```python
from build123d import *

# Parameters (mm, degrees)
F0_R     = 3
F0_W     = 10
F0_H     = 12
F1_DEPTH = 17
F2_R     = 3
F3_DEPTH = 12.5
F4_R     = 4


with BuildPart() as f1:
    # F0 (on Top) → F1 (new body)
    with BuildSketch(Plane.XY):
        with BuildLine():
            ThreePointArc((-12, -4), (-18, 2.0000000001), (-11.9999999997, 8))
            Line((-11.9999999997, 8), (-37.5, 8))
            Line((-37.5, 8), (-37.5, -4))
            Line((-37.5, -4), (-12, -4))
        make_face()
        with BuildLine():
            ThreePointArc((-6, 2), (-7.7573593128, 6.242640687), (-11.9999999997, 8))
            ThreePointArc((-11.9999999997, 8), (-18, 2.0000000001), (-12, -4))
            ThreePointArc((-12, -4), (-7.7573593129, -2.2426406871), (-6, 2))
        make_face()
        with Locations((-12, 2)):
            Circle(F0_R, mode=Mode.SUBTRACT)
        with Locations((-12, 2)):
            Circle(F0_R)
        with BuildLine():
            ThreePointArc((12, -4), (6, 2), (12, 8))
            Line((12, 8), (-11.9999999997, 8))
            ThreePointArc((-11.9999999997, 8), (-7.7573593128, 6.242640687), (-6, 2))
            ThreePointArc((-6, 2), (-7.7573593129, -2.2426406871), (-12, -4))
            Line((-12, -4), (12, -4))
        make_face()
        with BuildLine():
            ThreePointArc((12, -4), (16.2426406871, -2.2426406871), (18, 2))
            ThreePointArc((18, 2), (16.2426406871, 6.2426406871), (12, 8))
            ThreePointArc((12, 8), (6, 2), (12, -4))
        make_face()
        with Locations((12, 2)):
            Circle(F0_R, mode=Mode.SUBTRACT)
        with Locations((12, 2)):
            Circle(F0_R)
        with BuildLine():
            ThreePointArc((12, 8), (16.2426406871, 6.2426406871), (18, 2))
            ThreePointArc((18, 2), (16.2426406871, -2.2426406871), (12, -4))
            Line((12, -4), (37.5, -4))
            Line((37.5, -4), (37.5, 8))
            Line((37.5, 8), (12, 8))
        make_face()
        with Locations((-42.5, 2)):
            Rectangle(F0_W, F0_H)
        with Locations((42.5, 2)):
            Rectangle(F0_W, F0_H)
    extrude(amount=F1_DEPTH)

    # F2 (on Front) → F3 (cut, symmetric)
    with BuildSketch(Plane.XZ):
        with BuildLine():
            ThreePointArc((0, 9), (-3, 6), (0, 3))
            Line((0, 3), (0, 9))
        make_face()
        with BuildLine():
            Line((0, 9), (0, 3))
            ThreePointArc((0, 3), (2.1213203436, 3.8786796564), (3, 6))
            ThreePointArc((3, 6), (2.1213203436, 8.1213203436), (0, 9))
        make_face()
        with Locations((-27.4271778762, 6)):
            Circle(F2_R)
        with Locations((27.4271778762, 6)):
            Circle(F2_R)
    extrude(amount=F3_DEPTH, both=True, mode=Mode.SUBTRACT)

    # F4
    f4_edges = [f1.edges().sort_by_distance(p)[0] for p in [
        (-47.5, 2, 17),
        (47.5, 2, 17),
    ]]
    fillet(f4_edges, radius=F4_R)


solid = f1.part
```
Could you check a few things on this model? Use its own coordinates, in mm. Round coordinates to 2 decimals unless told otherwise and drop trailing zeros. Order: outer loops, then holes, each group sorted by start corner. A loop starts at its lowest first (then second) coordinate and runs counter-clockwise, first axis right, second up. Notation, with made-up numbers: (17.25, 21.25) -> (22.25, 21.25) arc R18 cw to (22.25, 36.25) -> close; hole circle Ø4 at (32.25, -26). An arc over 180 degrees is marked (long way). One line per question, with ' | ' between items.
Q1. If we section it at B-B on x = 29.5: Write out the boundary of the cut face in (y, z), plus the area to 3 significant figures.
Computed values:
outline: (-4, 0) -> (8, 0) -> (8, 3.83) -> (-4, 3.83) -> close; (-4, 8.17) -> (8, 8.17) -> (8, 17) -> (-4, 17) -> close | area: 152 mm²
Q2. If we section it at C-C on z = 15.5: Write out the boundary of the cut face in (x, y), plus the area to 3 significant figures.
Computed values:
outline: (-46.62, -4) -> (46.62, -4) -> (46.62, 8) -> (-46.62, 8) -> close | area: 1,120 mm²
Q3. We'd pull the mould along Z, two halves only. Please class faces 1 (the face through (1, 8, 10)), 2 (the face through (-1, 2, 0)), 3 (the face through (46.297, 2.084, 15.859)), 4 (the face through (24.43, 1.92, 6.13)): released by +Z, released by -Z, zero draft, split by the parting line, or undercut.
Computed values:
face 1: zero draft | face 2: released by -Z | face 3: released by +Z | face 4: undercut
Q4. If we section it at A-A on y = 4: Write out the boundary of the cut face in (x, z).
Computed values:
outline: (-47.5, 0) -> (47.5, 0) -> (47.5, 13) arc R4 ccw to (43.5, 17) -> (-43.5, 17) arc R4 ccw to (-47.5, 13) -> close; hole circle Ø6 at (-27.43, 6); hole circle Ø6 at (0, 6); hole circle Ø6 at (27.43, 6)
Q5. If I drill on line 1 (X direction, y = 4.75, z = 3.25); line 2 (Z direction, x = 28.5, y = -1); line 3 (Z direction, x = 1.5, y = 5.5), over which ranges is the centre line in solid material (lowest first)? Write a range as from..to.
Computed values:
line 1: -47.5..-28.63, -26.23..-1.2, 1.2..26.23, 28.63..47.5 | line 2: 0..3.2, 8.8..17 | line 3: 0..3.4, 8.6..17
